The listing builds one solid part. Answer for the finished solid, in the listing's coordinates (mm). Round coordinates to 2 decimals unless told otherwise and drop trailing zeros. Write each loop counter-clockwise with the first axis right and the second up, starting at its lowest first coordinate (ties: lowest second). Pieces come first, ordered by that corner, then holes. Notation, with made-up numbers: (28.5, 12) - (48.5, 12) arc R4 ccw to (48.5, 17) - close; hole circle Ø8 at (48.25, -26.5). An arc over 180 degrees is marked (long way). Return JSON: item names as keys, results as strings. Group by question number.
(1) Section A-A, the plane y = 2.5 is taken. Write down the section's boundary in (x, z), then the cut area to 3 significant figures.
(2) Section B-B, the plane z = -2 is taken. Write down the section's boundary in (x, y).
(3) Section D-D, the plane y = 0 is taken. Write down the section's boundary in (x, z).
(4) Each of these flat-tipped pins is pushed along its axis until it touches: pin 1 (3 mm diameter, centred on x = 6, y = 0.5, fed in from -Z); pin 2 (1.5 mm diameter, centred on x = 20, y = -2, fed in from +Z); pin 3 (1 mm diameter, centred on x = 24, y = 9, fed in from -Z); pin 4 (8 mm diameter, centred on x = 14, z = 3.5, fed in from -Y). Where does it stop, or does it pass through?
(5) Section C-C, the plane x = 24.5 is taken. Write down the section's boundary in (y, z).
(6) Determine the mould class of faces 1 (the cylindrical face through (32.047, -0.846, 6.445)), 2 (the flat face through (13.009, 5.381, -4.043)), 3 (the flat face through (0, 0, 11)), 4 (the cylindrical face through (30.206, -1.627, 12.394)) for opening direction Z: +Z half, -Z half, draft (parallel to the pull), parting line (faces both ways), or undercut.
(7) Find the intervals of material crossed by line 1 along Z through (x, y) = (40, 0); line 2 along Z through (x, y) = (14.5, 0), in increasing order. Write a range as [from, to].
```python
from build123d import *

# Parameters (mm, degrees)
F0_R          = 12.5
F1_DEPTH      = 50
F2_R          = 6.5
F3_DEPTH      = 50
F5_DEPTH      = 12.501
F5_DEPTH_BACK = 12.501


with BuildPart() as f1:
    # F0 (on Right) → F1 (new body)
    with BuildSketch(Plane.YZ):
        Circle(F0_R)
    extrude(amount=F1_DEPTH)

    # F2 (on face) → F3 (cut, through all)
    with BuildSketch(Plane.YZ.offset(50)):
        Circle(F2_R)
    extrude(amount=-F3_DEPTH, mode=Mode.SUBTRACT)

    # F4 (on Front) → F5 (cut, two sides)
    with BuildSketch(Plane.XZ) as f5_sk:
        Polygon((0, -12.5), (21.0457462817, -12.5), (0, 9.6463374794), align=None)
    extrude(amount=-F5_DEPTH, mode=Mode.SUBTRACT)
    extrude(f5_sk.sketch, amount=F5_DEPTH_BACK, mode=Mode.SUBTRACT)


solid = f1.part
```
Working result:
{
 "1": {"outline": "(0, 9.65) - (3.47, 6) - (50, 6) - (50, 12.25) - (0, 12.25) - close; (14.87, -6) - (20.81, -12.25) - (50, -12.25) - (50, -6) - close", "area": "507 mm^2"},
 "2": {"outline": "(11.07, -12.34) - (50, -12.34) - (50, -6.18) - (11.07, -6.18) - close; (11.07, 6.18) - (50, 6.18) - (50, 12.34) - (11.07, 12.34) - close"},
 "3": {"outline": "(0, 9.65) - (2.99, 6.5) - (50, 6.5) - (50, 12.5) - (0, 12.5) - close; (15.34, -6.5) - (21.05, -12.5) - (50, -12.5) - (50, -6.5) - close"},
 "4": {"pin 1": "stops at z = 6.18", "pin 2": "stops at z = 12.44", "pin 3": "stops at z = -9.17", "pin 4": "stops at y = -12.5"},
 "5": {"outline": "circle Ø25 at (0, 0); hole circle Ø13 at (0, 0)"},
 "6": {"face 1": "undercut", "face 2": "-Z half", "face 3": "draft", "face 4": "parting line"},
 "7": {"line 1": "z = [-12.5, -6.5], [6.5, 12.5]", "line 2": "z = [6.5, 12.5]"}
}
